For this review, take the finished solid that the model builds, in its own axes (mm). Face numbers are marked on the shaded views. A direction names the side the tool comes from. Round coordinates to 2 decimals unless told otherwise and drop trailing zeros. Loops run counter-clockwise (first coordinate to the right, second up) from the corner with the lowest first, then second, coordinate; pieces in that order, holes last.
1. To check wall thickness, follow line 1 along X through (y, z) = (7.75, 0); line 2 along Z through (x, y) = (-3, 7.75); line 3 along Y through (x, z) = (28, 9). State the ranges of each line that lie inside material, in increasing order.
2. Consider section A-A on y = 4.5. State the section outline as (x, z) points.
3. Clearance check with flat-ended pins moving along their axes: pin 1 Ø7 at (x, z) = (-1.5, 0) entering from +Y; pin 2 Ø7 at (x, z) = (-4.5, -3.5) entering from -Y; pin 3 Ø2 at (y, z) = (5.5, 11) entering from +X. State where each tip first meets the part, or that it passes through.
4. Draft analysis for pull direction Y (two halves, no side actions). For the marked faces 1, 2 and 3, state which applies: released by +Y, released by -Y, zero draft, split by the parting line, or undercut.
5. Tool access review of the marked faces 4 and 5: name each direction out of +Z, -Z, +X, -X, +Y, -Y from which nothing blocks a thin tool from reaching the whole face with its end or side.
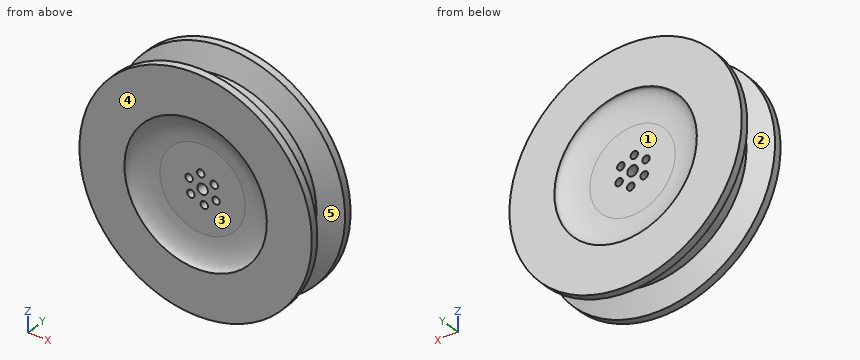
from build123d import *

# Parameters (mm, degrees)
SKETCH3_R          = 1
CUT_EXTRUDE1_DEPTH = 10


with BuildPart() as part:
    # Sketch2 → Revolve1 (revolve)
    with BuildSketch(Plane.XY, mode=Mode.PRIVATE) as revolve1_sk:
        with BuildLine():
            Line((-1.4, 9.635032461), (-1.4, 0.635032461))
            Line((-1.4, 0.635032461), (-11.4, 0.635032461))
            add(Edge.make_bspline(
                [(-11.4, 0.635032461), (-19, 0.635032461), (-19, -1.864967539)],
                knots=[4.71238898, 4.71238898, 4.71238898, 6.283185307, 6.283185307, 6.283185307], degree=2, weights=[1, 0.707106781, 1]))
            Line((-19, -1.864967539), (-31, -1.864967539))
            Line((-31, -1.864967539), (-31, 0.135032461))
            Line((-31, 0.135032461), (-25, 2.320032461))
            Line((-25, 2.320032461), (-25, 7.950032461))
            Line((-25, 7.950032461), (-31, 10.135032461))
            Line((-31, 10.135032461), (-31, 12.135032461))
            Line((-31, 12.135032461), (-19, 12.135032461))
            add(Edge.make_bspline(
                [(-19, 12.135032461), (-19, 9.635032461), (-11.4, 9.635032461)],
                knots=[0, 0, 0, 1.570796327, 1.570796327, 1.570796327], degree=2, weights=[1, 0.707106781, 1]))
            Line((-11.4, 9.635032461), (-1.4, 9.635032461))
        make_face()
    revolve(revolve1_sk.sketch.rotate(Axis((0, 6.223604304, 0), (0, -1, 0)), 270), axis=Axis((0, 6.223604304, 0), (0, -1, 0)))

    # Sketch3 → Cut-Extrude1 (cut)
    with BuildSketch(Plane(origin=(0, 9.635032461, 0), x_dir=(1, 0, 0), z_dir=(0, 1, 0))):
        with Locations(Location((-3.115047488, 2.346588832, 0), (0, 0, 270))):
            Circle(SKETCH3_R)
        with Locations(Location((0.474681797, 3.871004675, 0), (0, 0, 270))):
            Circle(SKETCH3_R)
        with Locations(Location((3.589729285, 1.524415842, 0), (0, 0, 270))):
            Circle(SKETCH3_R)
        with Locations(Location((3.115047488, -2.346588832, 0), (0, 0, 270))):
            Circle(SKETCH3_R)
        with Locations(Location((-0.474681797, -3.871004675, 0), (0, 0, 270))):
            Circle(SKETCH3_R)
        with Locations(Location((-3.589729285, -1.524415842, 0), (0, 0, 270))):
            Circle(SKETCH3_R)
    extrude(amount=-CUT_EXTRUDE1_DEPTH, mode=Mode.SUBTRACT)


solid = part.part
Resolved:
1. line 1: x = -25 to -1.4, 1.4 to 25
1. line 2: z = -24.82 to -3.34, -1.35 to 0.72, 2.33 to 24.82
1. line 3: y = -1.86 to 0.71, 9.56 to 12.14
2. outline: circle Ø50 at (0, 0); hole circle Ø2 at (-3.59, 1.52); hole circle Ø2 at (-3.12, -2.35); hole circle Ø2 at (-0.47, 3.87); hole circle Ø2.8 at (0, 0); hole circle Ø2 at (0.47, -3.87); hole circle Ø2 at (3.12, 2.35); hole circle Ø2 at (3.59, -1.52)
3. pin 1: stops at y = 9.64
3. pin 2: stops at y = 0.64
3. pin 3: stops at x = 22.91
4. face 1: released by +Y
4. face 2: undercut
4. face 3: released by -Y
5. face 4: +Z, -Z, +X, -X, -Y
5. face 5: none
